Model file for the job. Use its own axes, mm. Give positions to 0.01 mm unless a question says otherwise; leave off trailing zeros. Loops run counter-clockwise (first coordinate to the right, second up) from the corner with the lowest first, then second, coordinate; pieces in that order, holes last. Notation, with made-up numbers: M 52,51 L 99,51 A22 cw 99,77 Z; hole C 15,45.25 d7. An arc over 180 degrees is marked long. Answer in a Markdown table with one row per item.
Autodesk Inventor part; units mm, degrees
ref_plane "YZ Plane" through (0, 0, 0) normal (1, 0, 0) x (0, 1, 0)
ref_plane "XZ Plane" through (0, 0, 0) normal (0, 1, 0) x (-1, 0, 0)
ref_plane "XY Plane" through (0, 0, 0) normal (0, 0, 1) x (1, 0, 0)
sketch "Sketch1" plane through (0, 0, 0) normal (0, 1, 0) x (-1, 0, 0)
  circle A0 centre (0, 0) radius 53.34
  dimension "d0" = 106.68
extrude "Extrusion1" add sketch "Sketch1" along normal blind 2.54
sketch "Sketch2" plane through (0, 2.54, 0) normal (0, 1, 0) x (1, 0, 0)
  line L0 (0, 0) -> (33.676, 33.676) construction
  line L1 (0, 0) -> (47.625, 0) construction
  dimension "d3" = 47.625
  dimension "d4" = 45
hole "Hole1" at (33.676, 2.54, -33.676) direction (0, -1, 0) diameter 2.3876 end through all
pattern_circular "Circular Pattern1" count 6 over 360 about axis through (0, 0, 0) along (0, 1, 0) of "Hole1"
properties part number "4K shield cover" material "Brass, Soft Yellow"
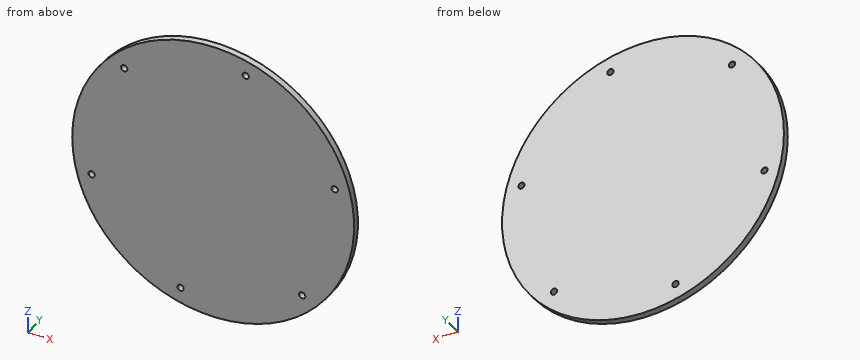
(1) Saw through at A-A, the plane y = 1.45. Give the cut face in (x, z), and give its area (3 significant figures).
Established:
| item | result |
|---|---|
| outline | C 0,0 d106.68; hole C -46,-12.33 d2.39; hole C -33.68,33.68 d2.39; hole C -12.33,-46 d2.39; hole C 12.33,46 d2.39; hole C 33.68,-33.68 d2.39; hole C 46,12.33 d2.39 |
| area | 8,910 mm2 |
(2) Saw through at B-B, the plane x = 39.5. Give the cut face in (y, z).
Established:
| item | result |
|---|---|
| outline | M 0,-35.85 L 2.54,-35.85 L 2.54,35.85 L 0,35.85 Z |
(3) Saw through at C-C, the plane z = -21.5. Give the cut face in (x, y).
Established:
| item | result |
|---|---|
| outline | M -48.82,0 L 48.82,0 L 48.82,2.54 L -48.82,2.54 Z |
(4) Wall check: L1, parallel to X at y = 0.7, z = -1; L2, parallel to Z at x = 47, y = 1.7; L3, parallel to X at y = 1.45, z = 33. Give the ranges that are in metal, low to high.
Established:
| item | result |
|---|---|
| L1 | x = -53.33 to 53.33 |
| L2 | z = -25.22 to 11.67, 12.98 to 25.22 |
| L3 | x = -41.91 to -34.66, -32.69 to 41.91 |
(5) Flat gauge pins, fed straight in: P1, Ø1.9, axis at x = 33.676, z = -33.676, coming from the -Y side; P2, Ø1, axis at y = 2, z = 1, coming from the -X side. Where does each tip first touch, or does it go through?
Established:
| item | result |
|---|---|
| P1 | passes through |
| P2 | stops at x = -53.34 |
